Source: CAD feature listing. Evaluate the final solid. Frame: model axes, mm. Give positions to 0.01 mm unless a question says otherwise; leave off trailing zeros. Order: outer loops, then holes, each group sorted by start corner. A loop starts at its lowest first (then second) coordinate and runs counter-clockwise, first axis right, second up.
from build123d import *

# Parameters (mm, degrees)
SKETCH7_W               = 4.7625
SKETCH7_H               = 2.12122512
BOSS_EXTRUDE2_DEPTH     = 130.175
SKETCH8_W               = 2.12122512
SKETCH8_H               = 4.7625
BOSS_EXTRUDE3_DEPTH     = 130.175
BOSS_EXTRUDE4_DEPTH     = 130.175
CUT_EXTRUDE6_DEPTH      = 245.098438966
CUT_EXTRUDE6_DEPTH_BACK = 245.098438966
CUT_EXTRUDE7_DEPTH      = 219.920809905
CUT_EXTRUDE7_DEPTH_BACK = 219.920809905


with BuildPart() as part:
    # Sketch7 → Boss-Extrude2 (new, symmetric)
    with BuildSketch(Plane.XY):
        with Locations((-4.92125, -2.560612608)):
            Rectangle(SKETCH7_W, SKETCH7_H)
    extrude(amount=BOSS_EXTRUDE2_DEPTH, both=True)

    # Sketch8 → Boss-Extrude3 (add, symmetric)
    with BuildSketch(Plane.XY):
        with Locations((-2.560612608, -4.92125)):
            Rectangle(SKETCH8_W, SKETCH8_H)
    extrude(amount=BOSS_EXTRUDE3_DEPTH, both=True)

    # Sketch11 → Boss-Extrude4 (add, symmetric)
    with BuildSketch(Plane.XY):
        with BuildLine():
            Line((-2.54, 1.500000048), (-2.54, -1.500000048))
            Line((-2.54, -1.500000048), (-7.3025, -1.500000048))
            Line((-7.3025, -1.500000048), (-7.3025, -3.621225168))
            Line((-7.3025, -3.621225168), (-5.866289198, -3.621225168))
            Line((-5.866289198, -3.621225168), (-3.621225168, -5.866289198))
            Line((-3.621225168, -5.866289198), (-3.621225168, -7.3025))
            Line((-3.621225168, -7.3025), (-1.500000048, -7.3025))
            Line((-1.500000048, -7.3025), (-1.500000048, -2.54))
            Line((-1.500000048, -2.54), (1.500000048, -2.54))
            Line((1.500000048, -2.54), (1.500000048, -0.519999976))
            ThreePointArc((1.500000048, -0.519999976), (0.908355739, 0.908355739), (-0.519999976, 1.500000048))
            Line((-0.519999976, 1.500000048), (-2.54, 1.500000048))
        make_face()
    extrude(amount=BOSS_EXTRUDE4_DEPTH, both=True)

    # Sketch18 → Cut-Extrude6 (cut, two sides)
    with BuildSketch(Plane(origin=(0, 0, 113.704878), x_dir=(-0.7071067811865466, 0.7071067811865485, 0), z_dir=(-0.5773502691896266, -0.577350269189625, -0.577350269189626))) as cut_extrude6_sk:
        Polygon((0, 0), (63.5, 36.661742094), (0, -73.323484187), (-63.5, 36.661742094), align=None)
    extrude(amount=CUT_EXTRUDE6_DEPTH, mode=Mode.SUBTRACT)
    extrude(cut_extrude6_sk.sketch, amount=-CUT_EXTRUDE6_DEPTH_BACK, mode=Mode.SUBTRACT)

    # Sketch19 → Cut-Extrude7 (cut, two sides)
    with BuildSketch(Plane(origin=(-66.606775424, -160.802980576, 0), x_dir=(0.7071067811865466, -0.7071067811865485, 0), z_dir=(0.7071067811865485, 0.7071067811865466, 0))) as cut_extrude7_sk:
        Polygon((-66.606775424, 0), (187.393224576, -254), (187.393224576, 254), (-320.606775424, 254), (-320.606775424, -254), align=None)
    extrude(amount=CUT_EXTRUDE7_DEPTH, mode=Mode.SUBTRACT)
    extrude(cut_extrude7_sk.sketch, amount=-CUT_EXTRUDE7_DEPTH_BACK, mode=Mode.SUBTRACT)

    # Sweep1: sweep along a curve in space
    with BuildLine() as sweep1_path:
        Line((-7.3025, -1.500000048, 4.102987064), (-2.54, -1.500000048, 0.735391018))
    # Sketch20 → Sweep1 (sweep)
    with BuildSketch(Plane.ZY.offset(2.54)):
        Polygon((4.906903198, 1.5), (4.906903198, -1.500000048), (0.735391018, -1.500000048), (2.85671143, 1.500000048), align=None)
    sweep(path=sweep1_path.line)

    # Sweep2: sweep along a curve in space
    with BuildLine() as sweep2_path:
        Line((-1.500000048, -2.54, 0.735391018), (-1.500000048, -7.3025, 4.102987064))
    # Sketch21 → Sweep2 (sweep)
    with BuildSketch(Plane.XZ.offset(2.54)):
        Polygon((-1.500000048, 4.906903198), (1.500000048, 4.906903198), (1.500000048, 2.85671143), (-1.500000048, 0.735391018), align=None)
    sweep(path=sweep2_path.line)


solid = part.part
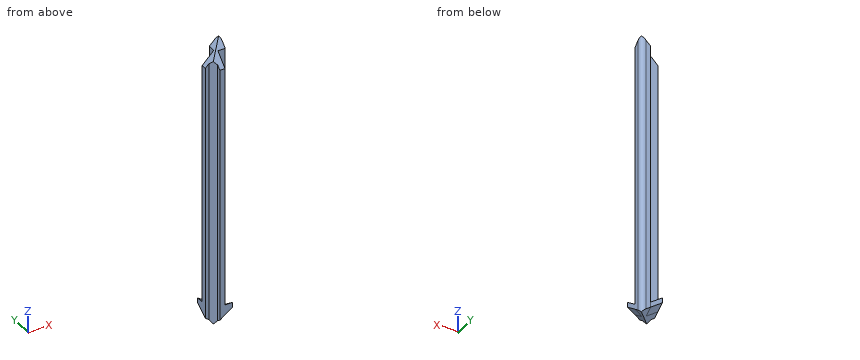
(1) Pin query (flat end, axial travel): pin 1 Ø2.5 at (y, z) = (0, 32.5) entering from -X; pin 2 Ø1.5 at (x, z) = (-0.5, 57) entering from -Y; pin 3 Ø1.5 at (y, z) = (-3.5, 71.5) entering from +X. Return the tip coordinate at first contact, or that it passes through.
(2) Line query: line 1 along X through (y, z) = (0, 33); line 2 along X through (y, z) = (-6.75, 92.5); line 3 along Y through (x, z) = (-3.25, 84). Output: solid intervals per line, ascending.
(3) Section A-A, the plane z = 14. Return loops of the section in (x, y).
Checks:
1. pin 1: stops at x = -2.54
1. pin 2: stops at y = -2.54
1. pin 3: stops at x = -1.5
2. line 1: x = -2.54 to 1.43
2. line 2: x = -3.62 to -1.5
2. line 3: y = -7.3 to -1.5
3. outline: (-7.3, -3.62) - (-5.87, -3.62) - (-3.62, -5.87) - (-3.62, -7.3) - (-1.5, -7.3) - (-1.5, -2.54) - (1.5, -2.54) - (1.5, -0.52) arc R2.02 ccw to (-0.52, 1.5) - (-2.54, 1.5) - (-2.54, -1.5) - (-7.3, -1.5) - close
